```python
from build123d import *

# Parameters (mm, degrees)
SKETCH1_W           = 50.8
SKETCH1_H           = 31.242
BOSS_EXTRUDE1_DEPTH = 1.27
BOSS_EXTRUDE2_DEPTH = 7.62
BOSS_EXTRUDE3_DEPTH = 5.08
SKETCH4_R           = 2.032
CUT_EXTRUDE1_DEPTH  = 7.62


with BuildPart() as part:
    # Sketch1 → Boss-Extrude1 (new body)
    with BuildSketch(Plane(origin=(0, 0, 0), x_dir=(1, 0, 0), z_dir=(0, 1, 0))):
        Rectangle(SKETCH1_W, SKETCH1_H)
    extrude(amount=BOSS_EXTRUDE1_DEPTH)

    # Sketch2 → Boss-Extrude2 (add)
    with BuildSketch(Plane(origin=(0, 1.27, 0), x_dir=(1, 0, 0), z_dir=(0, 1, 0))):
        Polygon((-25.4, 10.541), (-22.86, 10.541), (-22.86, 13.081), (-17.78, 13.081), (-17.78, 15.621), (-25.4, 15.621), align=None)
        Polygon((-25.4, -10.541), (-22.86, -10.541), (-22.86, -13.081), (-15.24, -13.081), (-15.24, -15.621), (-25.4, -15.621), align=None)
        Polygon((15.24, 15.621), (25.4, 15.621), (25.4, 5.461), (22.86, 5.461), (22.86, 13.081), (15.24, 13.081), align=None)
        Polygon((25.4, -5.461), (25.4, -15.621), (15.24, -15.621), (15.24, -13.081), (22.86, -13.081), (22.86, -5.461), align=None)
    extrude(amount=BOSS_EXTRUDE2_DEPTH)

    # Sketch3 → Boss-Extrude3 (add, symmetric)
    with BuildSketch(Plane(origin=(0, 0, 0), x_dir=(0, 0, -1), z_dir=(1, 0, 0))):
        Polygon((-13.081, 0), (-15.621, 0), (-15.621, 14.478), (-23.241, 14.478), (-23.241, 17.018), (-13.081, 17.018), align=None)
    boss_extrude3 = extrude(amount=BOSS_EXTRUDE3_DEPTH, both=True)

    # Sketch4 → Cut-Extrude1 (cut)
    with BuildSketch(Plane.XZ.offset(-14.478)):
        with Locations(Location((0, 19.431, 0), (0, 0, 270))):
            Circle(SKETCH4_R)
    cut_extrude1 = extrude(amount=-CUT_EXTRUDE1_DEPTH, mode=Mode.SUBTRACT)

    # Mirror2: Boss-Extrude3 across plane
    add(boss_extrude3.mirror(Plane.XY))

    # Mirror1: Cut-Extrude1 across plane
    add(cut_extrude1.mirror(Plane.XY), mode=Mode.SUBTRACT)


solid = part.part
```
The model under review builds one solid part; all positions refer to its coordinate system, in mm. A direction names the side the tool comes from. Round coordinates to 2 decimals unless told otherwise and drop trailing zeros. Loops run counter-clockwise (first coordinate to the right, second up) from the corner with the lowest first, then second, coordinate; pieces in that order, holes last. Notation, with made-up numbers: M 3.25,-15.5 L 37.25,-15.5 A18 cw 37.25,4.5 Z; hole C -15,39 d9. An arc over 180 degrees is marked long. Write item = value, one per line.
Item 1: Insertion check: P1, Ø6, axis at x = 18.5, y = 5, coming from the -Z side; P2, Ø5.5, axis at x = -20.5, y = 6, coming from the +Z side; P3, Ø4, axis at y = 5.5, z = 8, coming from the -X side. Each pin has a flat end and moves straight along its axis. Give the tip position at first contact, or say it passes through.
Return value:
P1 = -15.62
P2 = 15.62
P3 = 22.86
Item 2: For line 1 (Z direction, x = 21, y = 2); line 2 (Y direction, x = -0.5, z = 9.5); line 3 (X direction, y = 4, z = -7), list the stretches that pass through material, from the lowest coordinate up. Write a range as [from, to].
Return value:
line_1 = [-15.62, -13.08], [13.08, 15.62]
line_2 = [0, 1.27]
line_3 = [22.86, 25.4]
Item 3: Take a section at D-D on x = 12. Write out the cut boundary in (y, z), then the cut area to 3 significant figures.
Return value:
outline = M 0,-15.62 L 1.27,-15.62 L 1.27,15.62 L 0,15.62 Z
area = 39.7 mm2
Item 4: Take a section at C-C on z = 0. Write out the cut boundary in (x, y), then the cut area to 3 significant figures.
Return value:
outline = M -25.4,0 L 25.4,0 L 25.4,1.27 L -25.4,1.27 Z
area = 64.5 mm2
Item 5: Machinability: for faces 5 (the flat face through (-22.86, 5, -12)), 6 (the flat face through (-24, 5, 10.541)), 7 (the flat face through (-15.24, 5, 14)), 8 (the flat face through (2.3, 14.478, -19.4)), 9 (the flat face through (2.3, 14.478, 19.4)), which of the approach directions +Z, -Z, +X, -X, +Y, -Y give a long, thin tool a straight path to every point of the face, cutting with its end or side? Answer none if there is none.
Return value:
face_5 = +Y
face_6 = -X, +Y
face_7 = +Z, -Z, +Y
face_8 = -Z, +X, -X, -Y
face_9 = +Z, +X, -X, -Y
Item 6: Take a section at A-A on x = 0. Write out the cut boundary in (y, z), then the cut area to 3 significant figures.
Return value:
outline = M 0,-15.62 L 14.48,-15.62 L 14.48,-17.4 L 17.02,-17.4 L 17.02,-13.08 L 1.27,-13.08 L 1.27,13.08 L 17.02,13.08 L 17.02,17.4 L 14.48,17.4 L 14.48,15.62 L 0,15.62 Z; M 14.48,-23.24 L 17.02,-23.24 L 17.02,-21.46 L 14.48,-21.46 Z; M 14.48,21.46 L 17.02,21.46 L 17.02,23.24 L 14.48,23.24 Z
area = 138 mm2
Item 7: Take a section at B-B on x = -19. Write out the cut boundary in (y, z).
Return value:
outline = M 0,-15.62 L 8.89,-15.62 L 8.89,-13.08 L 1.27,-13.08 L 1.27,13.08 L 8.89,13.08 L 8.89,15.62 L 0,15.62 Z
Item 8: The part is to be moulded in two halves that separate along Z. For faces 1 (the flat face through (0, 0, 0)), 2 (the flat face through (-19, 5, 13.081)), 3 (the flat face through (0, 9, 13.081)), 4 (the flat face through (0, 6, -15.621)), say which applies: released by +Z, released by -Z, zero draft, split by the parting line, or undercut.
Return value:
face_1 = zero draft
face_2 = undercut
face_3 = undercut
face_4 = released by -Z
